Autodesk Inventor part; units mm, degrees
ref_plane "Work Plane3" through (0, 7.9375, 0) normal (0, 0.7071, 0.7071) x (-1, 0, 0)
ref_plane "YZ Plane" through (0, 0, 0) normal (1, 0, 0) x (0, 1, 0)
ref_plane "XY Plane" through (0, 0, 0) normal (0, 0, 1) x (1, 0, 0)
sketch "Sketch1" plane through (0, 0, 0) normal (0, 0, 1) x (1, 0, 0)
  circle A0 centre (0, 0) radius 7.9375
  dimension "d0" = 15.875
extrude "Extrusion1" add sketch "Sketch1" along normal blind 45.72
ref_plane "Work Plane2" through (0, 15.875, 0) normal (0, 1, 0) x (-1, 0, 0)
sketch "Sketch4" plane through (0, 15.875, 0) normal (0, 1, 0) x (-1, 0, 0)
  circle A0 centre (0, 7.62) radius 1.4605
  point P0 (0, 0)
  dimension "d6" = 2.921
  dimension "d7" = 7.62
sketch "Sketch5" plane through (0, 0, 0) normal (0, 0, -1) x (-1, 0, 0)
  circle A0 centre (0, 0) radius 7.9375
  circle A1 centre (0, 0.3175) radius 1.4605
  line L0 (0, 7.9375) -> (14.2875, 7.9375)
  dimension "d8" = 2.921
  dimension "d9" = 7.62
ref_plane "Work Plane3" through (0, 7.9375, 0) normal (0, 0.7071, 0.7071) x (-1, 0, 0)
sketch "Sketch6" plane through (0, 7.9375, 0) normal (0, 0.7071, 0.7071) x (-1, 0, 0)
  circle A0 centre (0, 3.9683) radius 1.5875
  point P0 (0, 5.6127)
  dimension "d11" = 3.175
extrude "Extrusion2" add sketch "Sketch6" along normal mid plane 25.4
sketch "Sketch7" plane through (0, -3.8488, -6.1742) normal (0, -0.7071, -0.7071) x (-1, 0, 0)
  circle A0 centre (0, 0) radius 1.5875
  circle A1 centre (0, 0) radius 1.5875
  point P0 (0, -1.6443)
hole "Hole1" at (-0.0004, -3.8478, -6.1752) direction (0, 0.7071, 0.7071) diameter 3.302 depth 25.4 tip angle 118
properties part number "Copper"
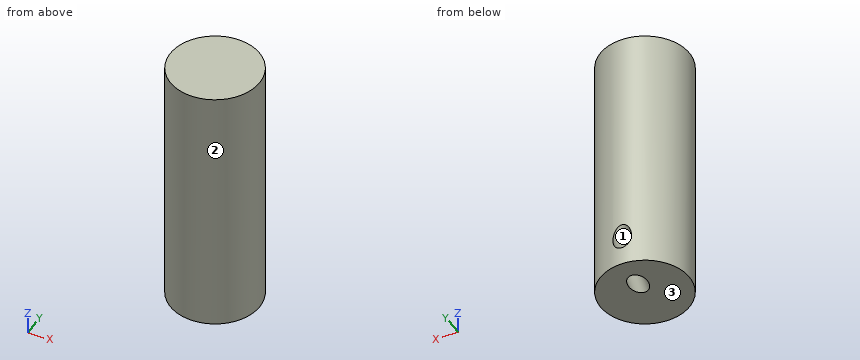
Design review of the part built by this model. Coordinates are the model's own, in mm. Face numbers are marked on the shaded views. Give positions to 0.01 mm unless a question says otherwise; leave off trailing zeros. Order: outer loops, then holes, each group sorted by start corner. A loop starts at its lowest first (then second) coordinate and runs counter-clockwise, first axis right, second up.
1. To check wall thickness, follow L1, parallel to Z at x = -1, y = 6.25; L2, parallel to X at y = 5, z = 3; L3, parallel to X at y = 7, z = 39. State the ranges of each line that lie inside material, in increasing order.
Solution:
L1: z = 0 to 2.06, 5.78 to 45.72
L2: x = -6.16 to -1.64, 1.63 to 6.16
L3: x = -3.74 to 3.74
2. Add section B-B, the plane z = 22.5. State the section outline as (x, y) points (1 decimal).
Solution:
outline: circle Ø15.9 at (0, 0)
3. Mouldability with a two-part tool opening along X and no side actions: class the marked faces 1, 2 and 3 as +X half, -X half, draft (parallel to the pull), parting line (faces both ways), or undercut.
Solution:
face 1: undercut
face 2: parting line
face 3: draft
4. Add section A-A, the plane x = 1. State the section outline as (y, z) points, then the cut area to 3 significant figures.
Solution:
outline: (-7.87, 0) - (0.47, 0) - (7.87, 7.4) - (7.87, 45.72) - (-7.87, 45.72) - close; (4.18, 0) - (7.87, 0) - (7.87, 3.69) - close
area: 699 mm2
5. For pin 1 Ø5 at (y, z) = (-5.5, 35.5) entering from +X; pin 2 Ø1.5 at (x, z) = (-4.5, 37.5) entering from +Y; pin 3 Ø2 at (y, z) = (6.5, 21.5) entering from +X, all flat-tipped, find the tip position at first contact; note any pin that passes through.
Solution:
pin 1: stops at x = 7.35
pin 2: stops at y = 7
pin 3: stops at x = 5.72
6. Add section D-D, the plane x = 7.25. State the section outline as (y, z) points.
Solution:
outline: (-3.23, 0) - (3.23, 0) - (3.23, 45.72) - (-3.23, 45.72) - close
7. Add section C-C, the plane y = -4. State the section outline as (x, z) points, then the cut area to 3 significant figures.
Solution:
outline: (-6.86, 0) - (6.86, 0) - (6.86, 45.72) - (-6.86, 45.72) - close
area: 627 mm2
